Design review of the part built by this model. Coordinates are the model's own, in mm. Face numbers are marked on the shaded views. Round coordinates to 2 decimals unless told otherwise and drop trailing zeros. Order: outer loops, then holes, each group sorted by start corner. A loop starts at its lowest first (then second) coordinate and runs counter-clockwise, first axis right, second up. Notation, with made-up numbers: M 47.25,74.25 L 105.25,74.25 A15 ccw 105.25,95.25 Z; hole C 72.25,62.25 d7. An arc over 180 degrees is marked long. Use a Markdown table: item, result. Add a question column.
(1) Take a section at D-D (y = 15). Write out the cut boundary in (x, z), then the cut area to 3 significant figures.
(2) Take a section at B-B (x = 19.5). Write out the cut boundary in (y, z), then the cut area to 3 significant figures.
(3) Take a section at A-A (x = 39). Write out the cut boundary in (y, z).
(4) To check wall thickness, follow probe 1 along X at (y, z) = (1.2, 8); probe 2 along Y at (x, z) = (32, 19). State the ranges of each line that lie inside material, in increasing order. Write a range as from..to.
(5) The part is to be moulded in two halves that separate along Y. For the marked faces 1, 2 and 3, say which applies: released by +Y, released by -Y, zero draft, split by the parting line, or undercut.
(6) Take a section at C-C (z = 14.95). Count the separate pieces of the cut face and the enclosed holes in it, then the cut area to 3 significant figures.
(7) For pin 1 (2 mm diameter, centred on y = 1.5, z = 2, fed in from -X); pin 2 (0.6 mm diameter, centred on x = 47.5, y = 1.5, fed in from +Z); pin 3 (1 mm diameter, centred on y = 1.5, z = 29.5, fed in from -X), all flat-tipped, find the tip position at first contact; note any pin that passes through.
```python
from build123d import *

# Parameters (mm, degrees)
SM_BASE_FLANGE_1_DEPTH   = 41
SKETCH_6_W               = 4
SKETCH_6_H               = 4
CUT_EXTRUDE_1_DEPTH      = 10
SKETCH_7_R               = 1.5
SKETCH_7_R_2             = 1.675
CUT_EXTRUDE_2_DEPTH      = 68.683085036
CUT_EXTRUDE_3_DEPTH      = 10
SKETCH_9_R               = 1.325
SKETCH_9_R_2             = 1.5
CUT_EXTRUDE_4_DEPTH      = 10
CUT_EXTRUDE_5_DEPTH      = 68.683085036
CUT_EXTRUDE_5_DEPTH_BACK = 68.683085036
SKETCH_10_W              = 7.72
SKETCH_10_H              = 10
CUT_EXTRUDE_6_DEPTH      = 68.683085036
CUT_EXTRUDE_6_DEPTH_BACK = 68.683085036
SKETCH_11_W              = 6
SKETCH_11_H              = 21.2
CUT_EXTRUDE_7_DEPTH      = 10
SKETCH_14_RX             = 3.175
SKETCH_14_RY             = 3
CUT_EXTRUDE_8_DEPTH      = 10
SKETCH_15_W              = 2.3
SKETCH_15_H              = 10
CUT_EXTRUDE_9_DEPTH      = 10
SKETCH_16_R              = 2.7
CUT_EXTRUDE_10_DEPTH     = 10
FILLET_1_R               = 2
SKETCH_17_R              = 1.325
CUT_EXTRUDE_11_DEPTH     = 10


# Sheet-metal steps are written as plain solids
with BuildPart() as part:
    # Sketch 1 → Базовая кромка1 (new body)
    with BuildSketch(Plane.XY):
        with BuildLine():
            Line((0, 22), (0, 4))
            ThreePointArc((0, 4), (1.171572875, 1.171572875), (4, 0))
            Line((4, 0), (50, 0))
            Line((50, 0), (50, 2))
            Line((50, 2), (4, 2))
            ThreePointArc((4, 2), (2.585786438, 2.585786438), (2, 4))
            Line((2, 4), (2, 22))
            Line((2, 22), (0, 22))
        make_face()
    extrude(amount=SM_BASE_FLANGE_1_DEPTH)

    # Эскиз6 → Вырез-Вытянуть1 (cut)
    with BuildSketch(Plane(origin=(0, 2, 0), x_dir=(1, 0, 0), z_dir=(0, 1, 0))):
        with Locations((48, -39)):
            Rectangle(SKETCH_6_W, SKETCH_6_H)
        with Locations((48, -2)):
            Rectangle(SKETCH_6_W, SKETCH_6_H)
    extrude(amount=-CUT_EXTRUDE_1_DEPTH, mode=Mode.SUBTRACT)

    # Эскиз7 → Вырез-Вытянуть2 (cut, through all)
    with BuildSketch(Plane(origin=(0, 2, 0), x_dir=(1, 0, 0), z_dir=(0, 1, 0))):
        with Locations(Location((39, -35, 0), (0, 0, 270))):
            Circle(SKETCH_7_R)
        with Locations(Location((39, -9, 0), (0, 0, 270))):
            Circle(SKETCH_7_R)
        with Locations(Location((41.975, -4.425, 0), (0, 0, 270))):
            Circle(SKETCH_7_R_2)
    extrude(amount=-CUT_EXTRUDE_2_DEPTH, mode=Mode.SUBTRACT)

    # Эскиз8 → Вырез-Вытянуть3 (cut)
    with BuildSketch(Plane(origin=(0, 2, 0), x_dir=(1, 0, 0), z_dir=(0, 1, 0))):
        with BuildLine():
            Line((34.75, -5.4), (30.25, -5.4))
            ThreePointArc((30.25, -5.4), (29, -4.15), (30.25, -2.9))
            Line((30.25, -2.9), (34.75, -2.9))
            ThreePointArc((34.75, -2.9), (36, -4.15), (34.75, -5.4))
        make_face()
        with BuildLine():
            Line((31.47, -8.3), (34.75, -8.3))
            ThreePointArc((34.75, -8.3), (36, -9.55), (34.75, -10.8))
            Line((34.75, -10.8), (31.47, -10.8))
            ThreePointArc((31.47, -10.8), (30.22, -9.55), (31.47, -8.3))
        make_face()
        with BuildLine():
            Line((31.25, -13.7), (34.75, -13.7))
            ThreePointArc((34.75, -13.7), (36, -14.95), (34.75, -16.2))
            Line((34.75, -16.2), (31.25, -16.2))
            ThreePointArc((31.25, -16.2), (30, -14.95), (31.25, -13.7))
        make_face()
        with BuildLine():
            Line((32.4, -19.1), (34.75, -19.1))
            ThreePointArc((34.75, -19.1), (36, -20.35), (34.75, -21.6))
            Line((34.75, -21.6), (32.4, -21.6))
            ThreePointArc((32.4, -21.6), (31.15, -20.35), (32.4, -19.1))
        make_face()
        with BuildLine():
            Line((31.05, -24.5), (34.75, -24.5))
            ThreePointArc((34.75, -24.5), (36, -25.75), (34.75, -27))
            Line((34.75, -27), (31.05, -27))
            ThreePointArc((31.05, -27), (29.8, -25.75), (31.05, -24.5))
        make_face()
        with BuildLine():
            Line((34.75, -32.4), (15.25, -32.4))
            ThreePointArc((15.25, -32.4), (14, -31.15), (15.25, -29.9))
            Line((15.25, -29.9), (34.75, -29.9))
            ThreePointArc((34.75, -29.9), (36, -31.15), (34.75, -32.4))
        make_face()
        with BuildLine():
            Line((15.25, -35.3), (34.75, -35.3))
            ThreePointArc((34.75, -35.3), (36, -36.55), (34.75, -37.8))
            Line((34.75, -37.8), (15.25, -37.8))
            ThreePointArc((15.25, -37.8), (14, -36.55), (15.25, -35.3))
        make_face()
    extrude(amount=-CUT_EXTRUDE_3_DEPTH, mode=Mode.SUBTRACT)

    # Эскиз9 → Вырез-Вытянуть4 (cut)
    with BuildSketch(Plane(origin=(0, 2, 0), x_dir=(1, 0, 0), z_dir=(0, 1, 0))):
        with Locations(Location((9.325, -36.475, 0), (0, 0, 270))):
            Circle(SKETCH_9_R)
        with Locations(Location((10.9, -28.85, 0), (0, 0, 270))):
            Circle(SKETCH_9_R_2)
        with Locations(Location((18.9, -8, 0), (0, 0, 270))):
            Circle(SKETCH_9_R_2)
    extrude(amount=-CUT_EXTRUDE_4_DEPTH, mode=Mode.SUBTRACT)

    # Эскиз10 → Вырез-Вытянуть5 (cut, two sides: drawn at the far end of the back side and taken through both)
    with BuildSketch(Plane(origin=(0, 2, 0), x_dir=(1, 0, 0), z_dir=(0, 1, 0)).offset(-CUT_EXTRUDE_5_DEPTH_BACK)):
        with Locations((3.86, -26.2)):
            Rectangle(SKETCH_10_W, SKETCH_10_H)
    extrude(amount=CUT_EXTRUDE_5_DEPTH + CUT_EXTRUDE_5_DEPTH_BACK, mode=Mode.SUBTRACT)

    # Эскиз11 → Вырез-Вытянуть6 (cut, two sides: drawn at the far end of the back side and taken through both)
    with BuildSketch(Plane(origin=(0, 2, 0), x_dir=(1, 0, 0), z_dir=(0, 1, 0)).offset(-CUT_EXTRUDE_6_DEPTH_BACK)):
        with Locations((3, -10.6)):
            Rectangle(SKETCH_11_W, SKETCH_11_H)
    extrude(amount=CUT_EXTRUDE_6_DEPTH + CUT_EXTRUDE_6_DEPTH_BACK, mode=Mode.SUBTRACT)

    # Эскиз12 → Вырез-Вытянуть7 (cut)
    with BuildSketch(Plane(origin=(0, 2, 0), x_dir=(1, 0, 0), z_dir=(0, 1, 0))):
        with BuildLine():
            Line((6, -3), (16, -3))
            Line((16, -3), (16, -8.028158581))
            ThreePointArc((16, -8.028158581), (16.344816391, -9.424582586), (17.3, -10.5))
            Line((17.3, -10.5), (17.3, -18))
            Line((17.3, -18), (20.6, -18))
            Line((20.6, -18), (20.6, -27.1))
            Line((20.6, -27.1), (13.6, -27.1))
            ThreePointArc((13.6, -27.1), (10.225833848, -25.703891292), (7.72, -28.36))
            Line((7.72, -28.36), (0.805596241, -28.36))
            Line((0.805596241, -28.36), (0.805596241, -3))
            Line((0.805596241, -3), (6, -3))
        make_face()
    extrude(amount=-CUT_EXTRUDE_7_DEPTH, mode=Mode.SUBTRACT)

    # Эскиз14 → Вырез-Вытянуть8 (cut)
    with BuildSketch(Plane(origin=(0, 2, 0), x_dir=(1, 0, 0), z_dir=(0, 1, 0))):
        with Locations(Location((26.3, -12.405), (0, 0, -90))):
            Ellipse(SKETCH_14_RX, SKETCH_14_RY)
    extrude(amount=-CUT_EXTRUDE_8_DEPTH, mode=Mode.SUBTRACT)

    # Эскиз15 → Вырез-Вытянуть9 (cut)
    with BuildSketch(Plane(origin=(0, 2, 0), x_dir=(1, 0, 0), z_dir=(0, 1, 0))):
        with Locations((26.3, -5)):
            Rectangle(SKETCH_15_W, SKETCH_15_H)
    extrude(amount=-CUT_EXTRUDE_9_DEPTH, mode=Mode.SUBTRACT)

    # Эскиз16 → Вырез-Вытянуть10 (cut)
    with BuildSketch(Plane(origin=(0, 2, 0), x_dir=(1, 0, 0), z_dir=(0, 1, 0))):
        with Locations(Location((26.1, -22.272936587, 0), (0, 0, 270))):
            Circle(SKETCH_16_R)
    extrude(amount=-CUT_EXTRUDE_10_DEPTH, mode=Mode.SUBTRACT)

    # Скругление1
    fillet_1_edges = [part.edges().sort_by_distance(p)[0] for p in [
        (1, 22, 31.2),
        (1, 22, 41),
    ]]
    fillet(fillet_1_edges, radius=FILLET_1_R)

    # Эскиз17 → Вырез-Вытянуть11 (cut)
    with BuildSketch(Plane.ZY):
        with Locations((36.1, 19.925)):
            Circle(SKETCH_17_R)
    extrude(amount=-CUT_EXTRUDE_11_DEPTH, mode=Mode.SUBTRACT)


solid = part.part
```
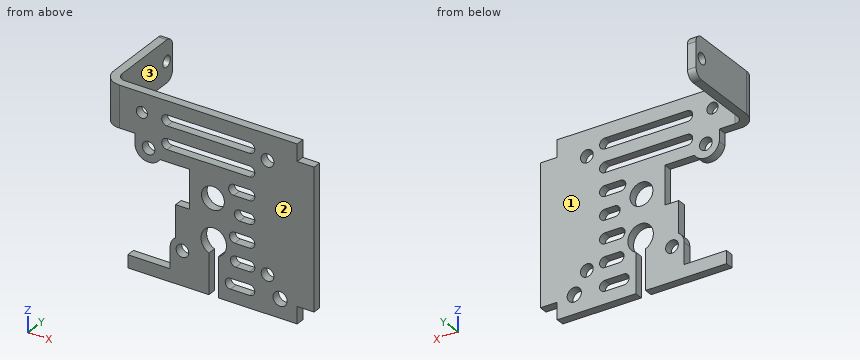
Verdict:
| question | item | result |
|---|---|---|
| 1 | outline | M 0,31.2 L 2,31.2 L 2,41 L 0,41 Z |
| 1 | area | 19.6 mm^2 |
| 2 | outline | M 0,0 L 2,0 L 2,6.63 L 0,6.63 Z; M 0,9.37 L 2,9.37 L 2,18 L 0,18 Z; M 0,27.1 L 2,27.1 L 2,29.9 L 0,29.9 Z; M 0,32.4 L 2,32.4 L 2,35.3 L 0,35.3 Z; M 0,37.8 L 2,37.8 L 2,41 L 0,41 Z |
| 2 | area | 48.3 mm^2 |
| 3 | outline | M 0,0 L 2,0 L 2,7.5 L 0,7.5 Z; M 0,10.5 L 2,10.5 L 2,33.5 L 0,33.5 Z; M 0,36.5 L 2,36.5 L 2,41 L 0,41 Z |
| 4 | probe 1 | x = 16..17.4, 20.4..25.15, 27.45..37.88, 40.12..50 |
| 4 | probe 2 | y = 0..2 |
| 5 | face 1 | released by +Y |
| 5 | face 2 | released by -Y |
| 5 | face 3 | zero draft |
| 6 | separate pieces | 3 |
| 6 | enclosed holes | 0 |
| 6 | area | 46.2 mm^2 |
| 7 | pin 1 | stops at x = 6 |
| 7 | pin 2 | stops at z = 37 |
| 7 | pin 3 | stops at x = 7.72 |
